```python
from build123d import *

# Parameters (mm, degrees)
SKETCH2_R           = 4.7625
BOSS_EXTRUDE1_DEPTH = 7.9375
SKETCH3_W           = 22.65
SKETCH3_H           = 2.54
SKETCH3_W_2         = 2.54
SKETCH3_H_2         = 23.525
EXTRUDE_THIN1_DEPTH = 2.54
FILLET1_R           = 1.5875


with BuildPart() as part:
    # Sketch1 → Revolve1 (revolve)
    with BuildSketch(Plane.XY, mode=Mode.PRIVATE) as revolve1_sk:
        with BuildLine():
            Line((-1.27, 25.4), (1.27, 25.4))
            Line((1.27, 25.4), (1.27, 27.6225))
            ThreePointArc((1.27, 27.6225), (0, 26.9875), (-1.27, 27.6225))
            Line((-1.27, 27.6225), (-1.27, 25.4))
        make_face()
    revolve(revolve1_sk.sketch.rotate(Axis((-2.168850248, 0, 0), (1, 0, 0)), 90), axis=Axis((-2.168850248, 0, 0), (1, 0, 0)))



with BuildPart() as body_2:
    # Sketch2 → Boss-Extrude1 (new body)
    with BuildSketch(Plane(origin=(1.27, 0, 0), x_dir=(0, 0, -1), z_dir=(1, 0, 0))):
        Circle(SKETCH2_R)
        with BuildLine():
            Line((-2.011684617, 1.875), (2.011684617, 1.875))
            ThreePointArc((2.011684617, 1.875), (2.75, 0), (2.011684617, -1.875))
            Line((2.011684617, -1.875), (-2.011684617, -1.875))
            ThreePointArc((-2.011684617, -1.875), (-2.75, 0), (-2.011684617, 1.875))
        make_face(mode=Mode.SUBTRACT)
    extrude(amount=-BOSS_EXTRUDE1_DEPTH)


with BuildPart() as part_1:
    add(part.part)

    add(body_2.part)  # Extrude-Thin1 merges body 2
    # Sketch3 → Extrude-Thin1 (add)
    with BuildSketch(Plane(origin=(1.27, 0, 0), x_dir=(0, 0, -1), z_dir=(1, 0, 0))):
        with Locations((-14.075, 0)):
            Rectangle(SKETCH3_W, SKETCH3_H)
        with Locations((0, 13.6375)):
            Rectangle(SKETCH3_W_2, SKETCH3_H_2)
        with Locations((14.075, 0)):
            Rectangle(SKETCH3_W, SKETCH3_H)
        with Locations((0, -13.6375)):
            Rectangle(SKETCH3_W_2, SKETCH3_H_2)
    extrude(amount=-EXTRUDE_THIN1_DEPTH)

    # Fillet1
    fillet1_edges = [part_1.edges().sort_by_distance(p)[0] for p in [
        (0, -1.27, -4.590044254),
        (0, -1.27, -25.368230131),
        (0, 1.27, 25.368230131),
        (0, -1.27, 25.368230131),
        (0, -4.590044254, -1.27),
        (0, -25.368230131, -1.27),
        (0, -4.590044254, 1.27),
        (0, -25.368230131, 1.27),
        (0, 1.27, 4.590044254),
        (0, -1.27, 4.590044254),
        (0, 25.368230131, 1.27),
        (0, 4.590044254, 1.27),
        (0, 4.590044254, -1.27),
        (0, 25.368230131, -1.27),
        (0, 1.27, -4.590044254),
        (0, 1.27, -25.368230131),
    ]]
    fillet(fillet1_edges, radius=FILLET1_R)


solid = part_1.part
```
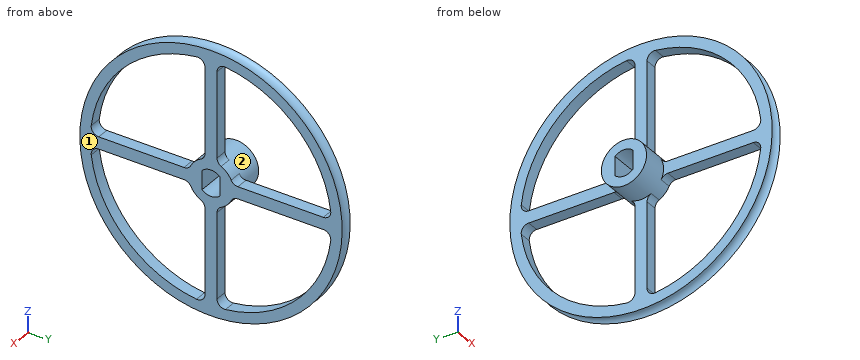
Design review of the part built by this model. Coordinates are the model's own, in mm. Face numbers are marked on the shaded views. A direction names the side the tool comes from. Round coordinates to 2 decimals unless told otherwise and drop trailing zeros. Write each loop counter-clockwise with the first axis right and the second up, starting at its lowest first coordinate (ties: lowest second). Pieces come first, ordered by that corner, then holes. Notation, with made-up numbers: (-8, -20) -> (0, -20) arc R26 ccw to (0, 13) -> close; hole circle Ø10 at (1.5, 57.5). An arc over 180 degrees is marked (long way). Write item = value, one per line. Start each with the question number.
1) Take a section at B-B, the plane z = 0. State the section outline as (x, y) points (1 decimal), plus the area to 3 significant figures.
2) Take a section at D-D, the plane y = 14.5. Count the separate pieces of the cut face and the enclosed holes in it, plus the area to 3 significant figures.
3) Clearance check with flat-ended pins moving along their axes: pin 1 (1.5 mm diameter, centred on x = -0.5, z = -19.5, fed in from -Y); pin 2 (0.8 mm diameter, centred on x = 0, z = 14, fed in from -Y); pin 3 (4.5 mm diameter, centred on x = -1.5, z = 0, fed in from -Y). State where each tip first meets the part, or that it passes through.
4) Wall thickness on probe 1 along Z at (x, y) = (-0.25, -13.5); probe 2 along Y at (x, z) = (0.25, -22); probe 3 along Y at (x, z) = (1, 20): over which ranges is each line inside the solid? List them lowest first. Write a range as from..to.
5) Tool access review of the marked faces 1 and 2: name each direction out of +Z, -Z, +X, -X, +Y, -Y from which nothing blocks a thin tool from reaching the whole face with its end or side.
Results list:
q1.outline = (-6.7, -4.8) -> (-1.3, -4.8) -> (-1.3, -27.6) arc R1.6 cw to (1.3, -27.6) -> (1.3, -1.9) -> (-6.7, -1.9) -> close; (-6.7, 1.9) -> (1.3, 1.9) -> (1.3, 27.6) arc R1.6 cw to (-1.3, 27.6) -> (-1.3, 4.8) -> (-6.7, 4.8) -> close
q1.area = 160 mm²
q2.separate_pieces = 3
q2.enclosed_holes = 0
q2.area = 17.3 mm²
q3.pin_1 = -19.74
q3.pin_2 = -23.31
q3.pin_3 = -27.62
q4.probe_1 = -23.39..-21.52, -1.27..1.27, 21.52..23.39
q4.probe_2 = -15.67..-12.69, -1.27..1.27, 12.69..15.67
q4.probe_3 = -18.64..-15.66, -1.27..1.27, 15.66..18.64
q5.face_1 = +Z, -Z, +X, +Y, -Y
q5.face_2 = -X
